Could you check a few things on this model? Use its own coordinates, in mm. A direction names the side the tool comes from. Give positions to 0.01 mm unless a question says otherwise; leave off trailing zeros. Order: outer loops, then holes, each group sorted by start corner. A loop starts at its lowest first (then second) coordinate and runs counter-clockwise, first axis right, second up. Notation, with made-up numbers: (46.5, -22.75) - (77.5, -22.75) arc R19 ccw to (77.5, 14.25) - close; hole circle Ø11 at (-15.5, 65.25). An arc over 180 degrees is marked (long way). Put each result on its own line as item: value.
from build123d import *

# Parameters (mm, degrees)
F0_W     = 127
F0_H     = 127
F1_DEPTH = 127
F2_W     = 88.9
F2_H     = 88.9
F3_DEPTH = 88.9
F4_R     = 25.4
F5_W     = 25.4
F5_H     = 25.4
F6_DEPTH = 38.1
F8_DEPTH = 38.1


with BuildPart() as f1:
    # F0 (on Front) → F1 (new body)
    with BuildSketch(Plane.XZ):
        with Locations((-63.5, 63.5)):
            Rectangle(F0_W, F0_H)
    extrude(amount=F1_DEPTH)

    # F2 (on face) → F3 (cut)
    with BuildSketch(Plane.XZ.offset(127)):
        with Locations((-44.45, 82.55)):
            Rectangle(F2_W, F2_H)
    extrude(amount=-F3_DEPTH, mode=Mode.SUBTRACT)

    # F4
    f4_edges = [f1.edges().sort_by_distance(p)[0] for p in [
        (0, -127, 19.05),
    ]]
    fillet(f4_edges, radius=F4_R)

    # F5 (on face) → F6 (cut)
    with BuildSketch(Plane.YZ.offset(-88.9)):
        with Locations((-82.55, 81.28)):
            Rectangle(F5_W, F5_H)
    extrude(amount=-F6_DEPTH, mode=Mode.SUBTRACT)

    # F7 (on face) → F8 (cut)
    with BuildSketch(Plane.XY.offset(38.1)):
        with BuildLine():
            ThreePointArc((-38.1, -81.28), (-70.620384, -67.809616), (-57.15, -100.33))
            ThreePointArc((-57.15, -100.33), (-43.679616, -94.750384), (-38.1, -81.28))
        make_face()
    extrude(amount=-F8_DEPTH, mode=Mode.SUBTRACT)


solid = f1.part
1) We'd pull the mould along Z, two halves only. Please class faces 4 (the flat face through (-99, -127, 50)), 5 (the flat face through (-35, -83, 38.1)), 6 (the flat face through (-108, -83, 93.98)): pulls with the +Z half, pulls with the -Z half, needs draft (parallel to the pull), parting line crosses it, or undercut.
Filled in:
face 4: needs draft
face 5: pulls with the +Z half
face 6: undercut
2) Which directions (+Z, -Z, +X, -X, +Y, -Y) give clear straight access to the entire face, cutting with the end or side of a thin tool? Please do faces 1 (the flat face through (-108, -95.25, 81)), 2 (the flat face through (-45, -38.1, 83)), 3 (the flat face through (0, -28, 48)).
Filled in:
face 1: +X, -X
face 2: +Z, +X, -Y
face 3: +Z, -Z, +X, +Y, -Y
3) Suppose I cut it at C-C, the plane z = 11.5. List the corners of the cut face in (x, y) for me, and give its area (3 significant figures).
Filled in:
outline: (-127, -127) - (-25.4, -127) arc R25.4 ccw to (0, -101.6) - (0, 0) - (-127, 0) - close; hole circle Ø38.1 at (-57.15, -81.28)
area: 14,900 mm^2
4) I'm going to push flat-ended pins straight in: pin 1 (4 mm diameter, centred on x = -76.5, z = 55, fed in from -Y); pin 2 (3 mm diameter, centred on x = -77, y = -63, fed in from +Z); pin 3 (8 mm diameter, centred on x = -93, z = 74.5, fed in from +Y). Where does each tip first touch, or does it pass through?
Filled in:
pin 1: stops at y = -38.1
pin 2: stops at z = 38.1
pin 3: stops at y = 0
5) Suppose I cut it at A-A, the plane z = 75. List the corners of the cut face in (x, y) for me.
Filled in:
outline: (-127, -127) - (-88.9, -127) - (-88.9, -95.25) - (-127, -95.25) - close; (-127, -69.85) - (-88.9, -69.85) - (-88.9, -38.1) - (0, -38.1) - (0, 0) - (-127, 0) - close
6) Suppose I cut it at B-B, the plane x = -99.5. List the corners of the cut face in (y, z) for me, and give its area (3 significant figures).
Filled in:
outline: (-127, 0) - (0, 0) - (0, 127) - (-127, 127) - close; hole (-95.25, 68.58) - (-69.85, 68.58) - (-69.85, 93.98) - (-95.25, 93.98) - close
area: 15,500 mm^2
7) Suppose I cut it at D-D, the plane x = -15. List the corners of the cut face in (y, z) for me, and give its area (3 significant figures).
Filled in:
outline: (-124.77, 0) - (0, 0) - (0, 127) - (-38.1, 127) - (-38.1, 38.1) - (-124.77, 38.1) - close
area: 8,140 mm^2
8) If I drill on line 1 (X direction, y = -81.28, z = 18.5); line 2 (X direction, y = -47, z = 71); line 3 (Y direction, x = -43, z = 94), over which ranges is the centre line in solid material (lowest first)? Write a range as [from, to].
Filled in:
line 1: x = [-127, -76.2], [-38.1, 0]
line 2: x = [-127, -88.9]
line 3: y = [-38.1, 0]
